```python
from build123d import *

# Parameters (mm, degrees)
SKETCH_1_R          = 6
SKETCH_1_R_2        = 2.55
EXTRUDE_1_DEPTH     = 5
SKETCH_2_R          = 2.55
EXTRUDE_2_DEPTH     = 5
FILLET_1_R          = 10
FILLET_2_R          = 5
SKETCH_3_R          = 1.25
CUT_EXTRUDE_1_DEPTH = 101.098617334


with BuildPart() as part:
    # ｽｹｯﾁ1 → ﾎﾞｽ - 押し出し1 (new body)
    with BuildSketch(Plane.XY):
        with BuildLine():
            Line((-40, -55), (40, -55))
            Line((40, -55), (40, -25))
            ThreePointArc((40, -25), (0, 15), (-40, -25))
            Line((-40, -25), (-40, -55))
        make_face()
        Circle(SKETCH_1_R, mode=Mode.SUBTRACT)
        with Locations((-30, -45)):
            Circle(SKETCH_1_R_2, mode=Mode.SUBTRACT)
        with Locations((0, -45)):
            Circle(SKETCH_1_R_2, mode=Mode.SUBTRACT)
        with Locations((30, -45)):
            Circle(SKETCH_1_R_2, mode=Mode.SUBTRACT)
    extrude(amount=EXTRUDE_1_DEPTH)

    # ｽｹｯﾁ2 → ﾎﾞｽ - 押し出し2 (add)
    with BuildSketch(Plane.XY.offset(5)):
        Polygon((-27.350889359, -92.947331922), (-40, -55), (-18.918148932, -55), (-8.377223398, -86.622776602), align=None)
        with Locations((-20.393878507, -82.195587877)):
            Circle(SKETCH_2_R, mode=Mode.SUBTRACT)
        with Locations((-25.137294997, -67.965338407)):
            Circle(SKETCH_2_R, mode=Mode.SUBTRACT)
    extrude(amount=-EXTRUDE_2_DEPTH)

    # ﾌｨﾚｯﾄ1
    fillet_1_edges = [part.edges().sort_by_distance(p)[0] for p in [
        (-18.918148932, -55, 2.5),
    ]]
    fillet(fillet_1_edges, radius=FILLET_1_R)

    # ﾌｨﾚｯﾄ2
    fillet_2_edges = [part.edges().sort_by_distance(p)[0] for p in [
        (-8.377223398, -86.622776602, 2.5),
        (-27.350889359, -92.947331922, 2.5),
        (40, -55, 2.5),
    ]]
    fillet(fillet_2_edges, radius=FILLET_2_R)

    # ｽｹｯﾁ3 → ｶｯﾄ - 押し出し1 (cut, through all)
    with BuildSketch(Plane.XY.offset(5)):
        with Locations((0, 11)):
            Circle(SKETCH_3_R)
        with Locations((9.526279442, -5.5)):
            Circle(SKETCH_3_R)
        with Locations((-9.526279442, -5.5)):
            Circle(SKETCH_3_R)
    extrude(amount=-CUT_EXTRUDE_1_DEPTH, mode=Mode.SUBTRACT)


solid = part.part
```
The listing builds one solid part. Answer for the finished solid, in the listing's coordinates (mm). A direction names the side the tool comes from. Coordinates: 2 decimals unless noted, no trailing zeros. Loops run counter-clockwise (first coordinate to the right, second up) from the corner with the lowest first, then second, coordinate; pieces in that order, holes last. Notation, with made-up numbers: (82, 88.5) -> (139, 88.5) arc R21 cw to (139, 117.5) -> close; hole circle Ø8 at (33.25, 86). An arc over 180 degrees is marked (long way). Return JSON: item names as keys, results as strings. Group by question number.
(1) Which of the six approach directions +Z, -Z, +X, -X, +Y, -Y give full straight-line access (tool end or side, diameter ignored) to faces 1 (the flat face through (15, -55, 2)), 2 (the cylindrical face through (-0.33, -42.47, 2.46)), 3 (the flat face through (-12.28, -74.92, 2.54))?
(2) A cutting plane is placed at C-C on y = 0. Write down the section's boundary in (x, z).
(3) Given pin 1 Ø1.5 at (x, y) = (0, 11) entering from -Z; pin 2 Ø2 at (x, z) = (-17.5, 4.5) entering from -Y; pin 3 Ø1.5 at (x, z) = (7.5, 2) entering from -Y, each flat-ended and moving along its own axis, determine where each tip first touches the part or whether it passes through.
(4) A cutting plane is placed at A-A on x = 0. Write down the section's boundary in (y, z), and give its area (3 significant figures).
(5) Find the intervals of material crossed by probe 1 along Y at (x, z) = (0, 2.05); probe 2 along X at (y, z) = (-46, 1.2); probe 3 along Y at (x, z) = (-1, 2.1), in increasing order. Write a range as from..to.
(6) Determine the mould class of faces 4 (the cylindrical face through (-27.017, -66.242, 2.535)), 5 (the cylindrical face through (-26.375, -91.119, 2.465)), 6 (the flat face through (40, -38, 2)) for opening direction X: released by +X, released by -X, zero draft, split by the parting line, or undercut.
(7) A cutting plane is placed at B-B on x = -30.5. Write down the section's boundary in (y, z).
(8) A cutting plane is placed at D-D on z = 0.95. Count the separate pieces of the cut face and the enclosed holes in it, and give its area (3 significant figures).
The answers:
{
 "1": {"face 1": "+Z, -Z, +X, -Y", "face 2": "+Z, -Z", "face 3": "+Z, -Z, +X"},
 "2": {"outline": "(-31.22, 0) -> (-6, 0) -> (-6, 5) -> (-31.22, 5) -> close; (6, 0) -> (31.22, 0) -> (31.22, 5) -> (6, 5) -> close"},
 "3": {"pin 1": "passes through", "pin 2": "stops at y = -90", "pin 3": "stops at y = -55"},
 "4": {"outline": "(-55, 0) -> (-47.55, 0) -> (-47.55, 5) -> (-55, 5) -> close; (-42.45, 0) -> (-6, 0) -> (-6, 5) -> (-42.45, 5) -> close; (6, 0) -> (9.75, 0) -> (9.75, 5) -> (6, 5) -> close; (12.25, 0) -> (15, 0) -> (15, 5) -> (12.25, 5) -> close", "area": "252 mm^2"},
 "5": {"probe 1": "y = -55..-47.55, -42.45..-6, 6..9.75, 12.25..15", "probe 2": "x = -40..-32.35, -27.65..-2.35, 2.35..27.65, 32.35..40", "probe 3": "y = -55..-47.35, -42.65..-5.92, 5.92..10.25, 11.75..14.99"},
 "6": {"face 4": "undercut", "face 5": "split by the parting line", "face 6": "released by +X"},
 "7": {"outline": "(-83.5, 0) -> (-47.5, 0) -> (-47.5, 5) -> (-83.5, 5) -> close; (-42.5, 0) -> (0.88, 0) -> (0.88, 5) -> (-42.5, 5) -> close"},
 "8": {"separate pieces": "1", "enclosed holes": "9", "area": "5,440 mm^2"}
}
